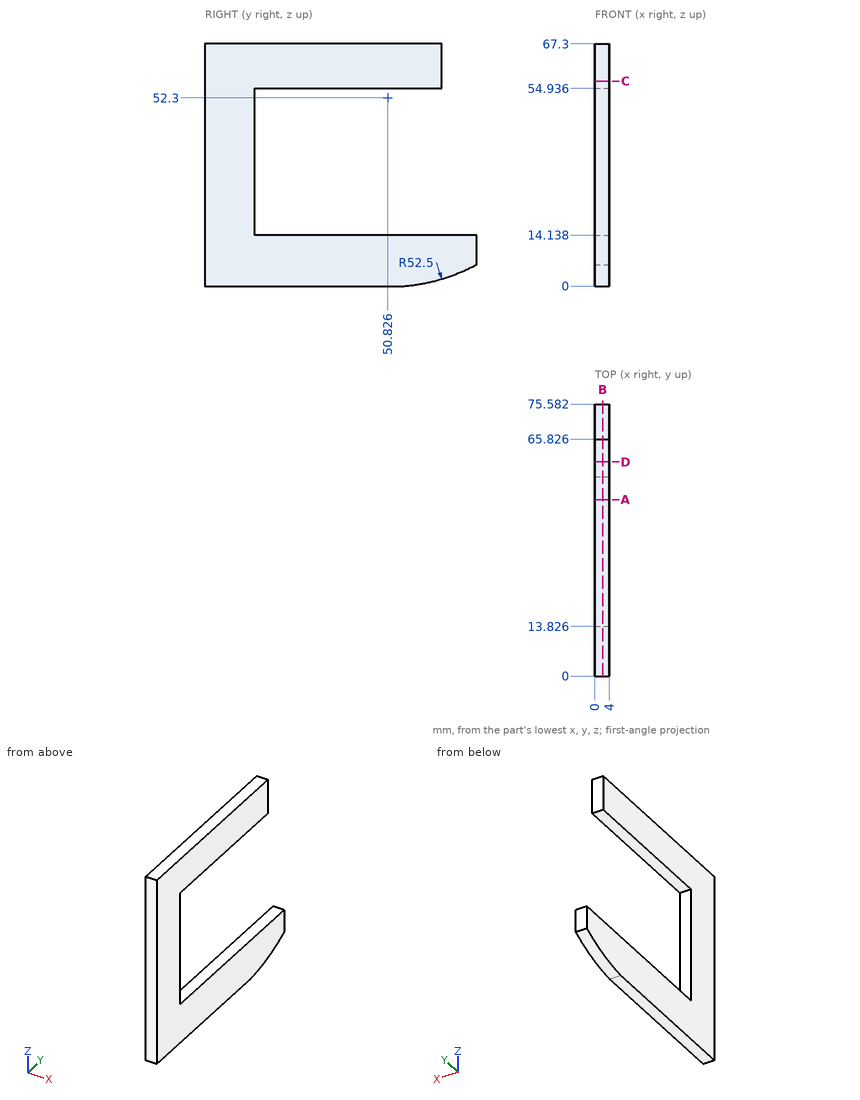
Could you check a few things on this drawing? It's one solid part, dimensions in mm from its lowest x, y, z. Give positions to 0.01 mm unless a question says otherwise; leave off trailing zeros. Write each loop counter-clockwise with the first axis right and the second up, starting at its lowest first coordinate (ties: lowest second). Pieces come first, ordered by that corner, then holes.
(1) Imagine slicing it at A-A, the plane y = 49. Write out the boundary of the cut face in (x, z), and give its area (3 significant figures).
Output values:
outline: (0, 0) - (4, 0) - (4, 14.14) - (0, 14.14) - close; (0, 54.94) - (4, 54.94) - (4, 67.3) - (0, 67.3) - close
area: 106 mm2
(2) If I drill on L1, parallel to Z at x = 3.6, y = 14.5; L2, parallel to Y at x = 0.95, z = 41; L3, parallel to Y at x = 3.2, z = 64, over which ranges is the centre line in solid material (lowest first)?
Output values:
L1: z = 0 to 14.14, 54.94 to 67.3
L2: y = 0 to 13.83
L3: y = 0 to 65.83
(3) Imagine slicing it at B-B, the plane x = 2.2. Write out the boundary of the cut face in (y, z) (1 decimal).
Output values:
outline: (0, 0) - (55.4, 0) arc R52.5 ccw to (75.6, 6) - (75.6, 14.1) - (13.8, 14.1) - (13.8, 54.9) - (65.8, 54.9) - (65.8, 67.3) - (0, 67.3) - close
(4) Will these pins go through, and if not, where does the flat tip stop? pin 1 (2 mm diameter, centred on x = 2, z = 24, fed in from +Y); pin 2 (8 mm diameter, centred on y = 21, z = 39.5, fed in from +X); pin 3 (1 mm diameter, centred on x = 0.5, z = 54, fed in from -Y).
Output values:
pin 1: stops at y = 13.83
pin 2: passes through
pin 3: stops at y = 0
(5) Imagine slicing it at C-C, the plane z = 57. Write out the boundary of the cut face in (x, y).
Output values:
outline: (0, 0) - (4, 0) - (4, 65.83) - (0, 65.83) - close
(6) Imagine slicing it at D-D, the plane y = 59.5. Write out the boundary of the cut face in (x, z).
Output values:
outline: (0, 0.52) - (4, 0.52) - (4, 14.14) - (0, 14.14) - close; (0, 54.94) - (4, 54.94) - (4, 67.3) - (0, 67.3) - close
